Answer from the drawing. Dimensions are ordinates in mm from the lowest x, y and z of the part. A direction names the side the tool comes from. Give positions to 0.01 mm unless a question says otherwise; leave off trailing zeros. Write each loop counter-clockwise with the first axis right and the second up, starting at its lowest first coordinate (ties: lowest second). Pieces come first, ordered by that corner, then holes.
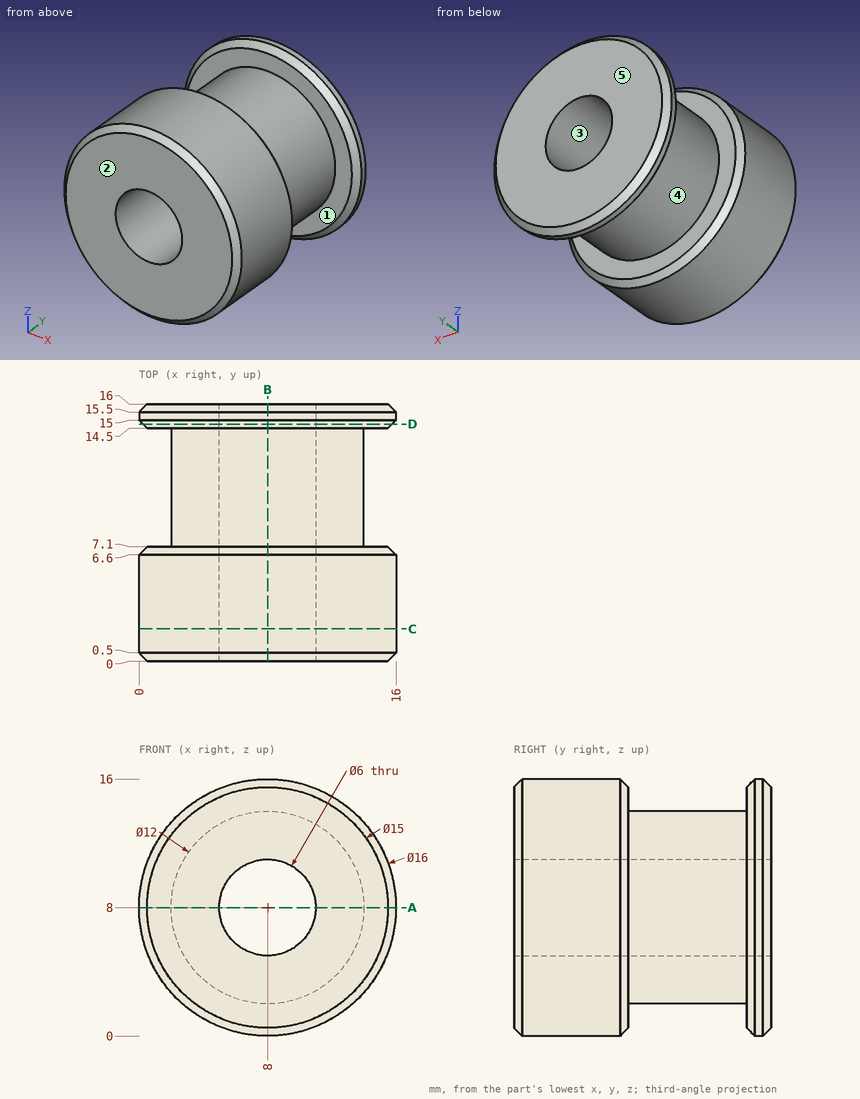
Item 1: Find the intervals of material crossed by line 1 along Z through (x, y) = (8, 11.5); line 2 along Z through (x, y) = (8, 4); line 3 along Y through (x, z) = (9, 14), in increasing order.
Result set:
line 1: z = 2 to 5, 11 to 14
line 2: z = 0 to 5, 11 to 16
line 3: y = 0 to 7.1, 14.5 to 16
Item 2: Section A-A (z = 8) is taken. Write down the section's boundary in (x, y), and give its area (3 significant figures).
Result set:
outline: (0, 0.5) - (0.5, 0) - (5, 0) - (5, 16) - (0.5, 16) - (0, 15.5) - (0, 15) - (0.5, 14.5) - (2, 14.5) - (2, 7.1) - (0.5, 7.1) - (0, 6.6) - close; (11, 0) - (15.5, 0) - (16, 0.5) - (16, 6.6) - (15.5, 7.1) - (14, 7.1) - (14, 14.5) - (15.5, 14.5) - (16, 15) - (16, 15.5) - (15.5, 16) - (11, 16) - close
area: 129 mm2
Item 3: Section B-B (x = 8) is taken. Write down the section's boundary in (y, z).
Result set:
outline: (0, 0.5) - (0.5, 0) - (6.6, 0) - (7.1, 0.5) - (7.1, 2) - (14.5, 2) - (14.5, 0.5) - (15, 0) - (15.5, 0) - (16, 0.5) - (16, 5) - (0, 5) - close; (0, 11) - (16, 11) - (16, 15.5) - (15.5, 16) - (15, 16) - (14.5, 15.5) - (14.5, 14) - (7.1, 14) - (7.1, 15.5) - (6.6, 16) - (0.5, 16) - (0, 15.5) - close
Item 4: Which of the six approach directions +Z, -Z, +X, -X, +Y, -Y give full straight-line access (tool end or side, diameter ignored) to the marked faces 1 and 2?
Result set:
face 1: none
face 2: +Z, -Z, +X, -X, -Y
Item 5: Section D-D (y = 14.75) is taken. Write down the section's boundary in (x, z).
Result set:
outline: circle Ø15.5 at (8, 8); hole circle Ø6 at (8, 8)
Item 6: Section C-C (y = 2) is taken. Write down the section's boundary in (x, z).
Result set:
outline: circle Ø16 at (8, 8); hole circle Ø6 at (8, 8)
Item 7: Each of these flat-tipped pins is pushed along its axis until it touches: pin 1 Ø4 at (x, y) = (5, 13) entering from +Z (3 decimals); pin 2 Ø1.5 at (x, y) = (9.5, 8) entering from +Z; pin 3 Ø2 at (y, z) = (5, 6.5) entering from -X. Where does it stop, or does it pass through?
Result set:
pin 1: stops at z = 15.535
pin 2: stops at z = 13.95
pin 3: stops at x = 0.02
Item 8: Determine the mould class of the marked faces 3, 4 and 5 for opening direction Y: pulls with the +Y half, pulls with the -Y half, needs draft (parallel to the pull), parting line crosses it, or undercut.
Result set:
face 3: needs draft
face 4: undercut
face 5: pulls with the +Y half
